Autodesk Inventor part; units mm, degrees
ref_plane "YZ Plane" through (0, 0, 0) normal (1, 0, 0) x (0, 1, 0)
ref_plane "XZ Plane" through (0, 0, 0) normal (0, 1, 0) x (-1, 0, 0)
ref_plane "XY Plane" through (0, 0, 0) normal (0, 0, 1) x (1, 0, 0)
sketch "Sketch1" plane through (0, 0, 0) normal (0, 0, 1) x (1, 0, 0)
  line L0 (0, 0) -> (50, 0)
  line L1 (50, 0) -> (50, 255.203)
  line L2 (50, 255.203) -> (0, 255.203)
  line L3 (0, 255.203) -> (0, 0)
  dimension "d0" = 50
  dimension "d1" = 255.203
extrude "Extrusion1" add sketch "Sketch1" along normal blind 5
sketch "Sketch2" plane through (0, 0, 0) normal (0, -1, 0) x (1, 0, 0)
  line L0 (36.5, 2.5) -> (13.5, 2.5) construction
  line L1 (36.5, 3.5) -> (13.5, 3.5)
  line L2 (13.5, 1.5) -> (36.5, 1.5)
  arc A0 (36.5, 1.5) -> (36.5, 3.5) centre (36.5, 2.5) ccw
  arc A1 (13.5, 3.5) -> (13.5, 1.5) centre (13.5, 2.5) ccw
  line L3 (50, 0) -> (50, 5)
  point P0 (0, 0)
  point P1 (25, 2.5)
  point P2 (50, 2.5)
  point P3 (12.5, 2.5)
  point P4 (37.5, 2.5)
  dimension "d4" = 2
  dimension "d5" = 25
  dimension "d6" = 25
  dimension "d9" = 2.5
extrude "Extrusion2" add sketch "Sketch2" along normal blind 10
sketch "Sketch3" plane through (0, 255.203, 0) normal (0, 1, 0) x (1, 0, 0)
  line L0 (36.5, -2.5) -> (13.5, -2.5) construction
  line L1 (36.5, -1.5) -> (13.5, -1.5)
  line L2 (13.5, -3.5) -> (36.5, -3.5)
  arc A0 (36.5, -3.5) -> (36.5, -1.5) centre (36.5, -2.5) ccw
  arc A1 (13.5, -1.5) -> (13.5, -3.5) centre (13.5, -2.5) ccw
  point P0 (0, 0)
  point P1 (25, -2.5)
  point P2 (12.5, -2.5)
  point P3 (37.5, -2.5)
  dimension "d10" = 2
  dimension "d12" = 25
  dimension "d14" = 2.5
  dimension "d15" = 25
extrude "Extrusion3" add sketch "Sketch3" along normal blind 10
Verification items for the finished model (mm, model axes). A direction names the side the tool comes from. Coordinates: 2 decimals unless noted, no trailing zeros. Write each loop counter-clockwise with the first axis right and the second up, starting at its lowest first coordinate (ties: lowest second). Pieces come first, ordered by that corner, then holes. Notation, with made-up numbers: (-6, -5.75) - (28, -5.75) arc R30 ccw to (28, 16.25) - close; hole circle Ø6 at (37.25, 49). An arc over 180 degrees is marked (long way). Write item = value, one per line.
Q1. Material ranges on L1, parallel to Y at x = 27.5, z = 4.1, recorded low to high. Write a range as from..to.
Answer:
L1 = 0..255.2
Q2. Cross-section at B-B (z = 2.5). Enter the section's corners in (x, y).
Answer:
outline = (0, 0) - (12.5, 0) - (12.5, -10) - (37.5, -10) - (37.5, 0) - (50, 0) - (50, 255.2) - (37.5, 255.2) - (37.5, 265.2) - (12.5, 265.2) - (12.5, 255.2) - (0, 255.2) - close
Q3. Access from +Z, -Z, +X, -X, +Y, -Y to the whole of each face (thin tool, end or side, straight path). Record for faces 4 (the face through (50, 126, 2)), 5 (the face through (25, -5, 1.5)), 6 (the face through (25, -5, 3.5)).
Answer:
face_4 = +Z, -Z, +X, +Y, -Y
face_5 = -Z, +X, -X, -Y
face_6 = +Z, +X, -X, -Y
Q4. Cross-section at C-C (x = 41.5). Enter the section's corners in (y, z), plus the area to 3 significant figures.
Answer:
outline = (0, 0) - (255.2, 0) - (255.2, 5) - (0, 5) - close
area = 1,280 mm²
Q5. Cross-section at A-A (x = 21). Enter the section's corners in (y, z), plus the area to 3 significant figures.
Answer:
outline = (-10, 1.5) - (0, 1.5) - (0, 0) - (255.2, 0) - (255.2, 1.5) - (265.2, 1.5) - (265.2, 3.5) - (255.2, 3.5) - (255.2, 5) - (0, 5) - (0, 3.5) - (-10, 3.5) - close
area = 1,320 mm²
Q6. Go/stop test with flat-tipped pins: pin 1 Ø10 at (x, y) = (43, 145) entering from -Z; pin 2 Ø5 at (x, y) = (21.5, -7) entering from -Z; pin 3 Ø11 at (x, y) = (26, -6) entering from +Z. Record where each tip stops, or that it passes through.
Answer:
pin_1 = 0
pin_2 = 1.5
pin_3 = 3.5
Q7. Mould release check, pull along Z, two halves, no side actions. Record for faces 1 (the face through (25, 255.203, 1)), 2 (the face through (25, 260, 1.5)), 3 (the face through (25, 260, 3.5)): released by +Z, released by -Z, zero draft, split by the parting line, or undercut.
Answer:
face_1 = zero draft
face_2 = released by -Z
face_3 = released by +Z
